```python
from build123d import *

# Parameters (mm, degrees)
SKETCH1_W           = 100
SKETCH1_H           = 154
SKETCH1_R           = 2
BOSS_EXTRUDE1_DEPTH = 5


with BuildPart() as part:
    # Sketch1 → Boss-Extrude1 (new body)
    with BuildSketch(Plane(origin=(0, 0, 0), x_dir=(1, 0, 0), z_dir=(0, 1, 0))):
        with Locations((23.349056604, 51.646226415)):
            Rectangle(SKETCH1_W, SKETCH1_H)
        with Locations(Location((-6.650943396, 73.646226415, 0), (0, 0, 270))):
            Circle(SKETCH1_R, mode=Mode.SUBTRACT)
        with Locations(Location((-6.650943396, 29.646226415, 0), (0, 0, 90))):
            Circle(SKETCH1_R, mode=Mode.SUBTRACT)
        with BuildLine():
            Line((45.849056604, 79.646226415), (60.849056604, 79.646226415))
            ThreePointArc((60.849056604, 79.646226415), (63.849056604, 76.646226415), (60.849056604, 73.646226415))
            Line((60.849056604, 73.646226415), (45.849056604, 73.646226415))
            ThreePointArc((45.849056604, 73.646226415), (42.849056604, 76.646226415), (45.849056604, 79.646226415))
        make_face(mode=Mode.SUBTRACT)
        with BuildLine():
            Line((10.849056604, 54.646226415), (25.849056604, 54.646226415))
            ThreePointArc((25.849056604, 54.646226415), (28.849056604, 51.646226415), (25.849056604, 48.646226415))
            Line((25.849056604, 48.646226415), (10.849056604, 48.646226415))
            ThreePointArc((10.849056604, 48.646226415), (7.849056604, 51.646226415), (10.849056604, 54.646226415))
        make_face(mode=Mode.SUBTRACT)
        with BuildLine():
            Line((45.849056604, 29.646226415), (60.849056604, 29.646226415))
            ThreePointArc((60.849056604, 29.646226415), (63.849056604, 26.646226415), (60.849056604, 23.646226415))
            Line((60.849056604, 23.646226415), (45.849056604, 23.646226415))
            ThreePointArc((45.849056604, 23.646226415), (42.849056604, 26.646226415), (45.849056604, 29.646226415))
        make_face(mode=Mode.SUBTRACT)
    extrude(amount=BOSS_EXTRUDE1_DEPTH)


solid = part.part
```
Geometry check sheet. Reference: the model listing, model coordinates, mm. A direction names the side the tool comes from. Coordinates: 2 decimals unless noted, no trailing zeros. Write each loop counter-clockwise with the first axis right and the second up, starting at its lowest first coordinate (ties: lowest second). Pieces come first, ordered by that corner, then holes. Notation, with made-up numbers: M -19,34 L 31,34 A22 ccw 31,66 Z; hole C -30,-9.5 d4. An arc over 180 degrees is marked long. Answer as a JSON object with one key per item and string values.
1. Section check C-C, the plane y = 3. Enter the section's corners in (x, z), plus the area to 3 significant figures.
Answers below:
{"outline": "M -26.65,-128.65 L 73.35,-128.65 L 73.35,25.35 L -26.65,25.35 Z; hole C -6.65,-73.65 d4; hole C -6.65,-29.65 d4; hole M 10.85,-54.65 L 25.85,-54.65 A3 ccw 25.85,-48.65 L 10.85,-48.65 A3 ccw Z; hole M 45.85,-79.65 L 60.85,-79.65 A3 ccw 60.85,-73.65 L 45.85,-73.65 A3 ccw Z; hole M 45.85,-29.65 L 60.85,-29.65 A3 ccw 60.85,-23.65 L 45.85,-23.65 A3 ccw Z", "area": "15,000 mm²"}
2. Draft check along X on faces 1 (the flat face through (-26.651, 2, -51)), 2 (the flat face through (23, 2, -128.646)), 3 (the cylindrical face through (63.85, 2.46, -26.71)). Enter one of: released by +X, released by -X, zero draft, split by the parting line, or undercut.
Answers below:
{"face 1": "released by -X", "face 2": "zero draft", "face 3": "undercut"}
3. Section check A-A, the plane x = 22. Enter the section's corners in (y, z), plus the area to 3 significant figures.
Answers below:
{"outline": "M 0,-128.65 L 5,-128.65 L 5,-54.65 L 0,-54.65 Z; M 0,-48.65 L 5,-48.65 L 5,25.35 L 0,25.35 Z", "area": "740 mm²"}
4. Tool access check on faces 4 (the flat face through (53, 2, -23.646)), 5 (the flat face through (23, 2, 25.354)). Record the directions out of +Z, -Z, +X, -X, +Y, -Y that give a thin tool (end or side, any length) a straight path to the whole face; none if there is none.
Answers below:
{"face 4": "+Y, -Y", "face 5": "+Z, +X, -X, +Y, -Y"}
5. Go/stop test with a flat-tipped pin: pin 1 Ø4.5 at (x, z) = (-6.65, -29.65) entering from -Y. Record where the tip stops, or that it passes through.
Answers below:
{"pin 1": "stops at y = 0"}
6. Section check B-B, the plane x = 57. Enter the section's corners in (y, z), plus the area to 3 significant figures.
Answers below:
{"outline": "M 0,-128.65 L 5,-128.65 L 5,-79.65 L 0,-79.65 Z; M 0,-73.65 L 5,-73.65 L 5,-29.65 L 0,-29.65 Z; M 0,-23.65 L 5,-23.65 L 5,25.35 L 0,25.35 Z", "area": "710 mm²"}
7. Scan lines: L1, parallel to Z at x = 59, y = 3.85; L2, parallel to Z at x = 12.5, y = 0.75; L3, parallel to Z at x = 26, y = 1.1. Record each from-to range of solid material in increasing order.
Answers below:
{"L1": "z = -128.65 to -79.65, -73.65 to -29.65, -23.65 to 25.35", "L2": "z = -128.65 to -54.65, -48.65 to 25.35", "L3": "z = -128.65 to -54.64, -48.65 to 25.35"}
